Check sheet for the modelled part. Datum: model origin and axes. Units: mm. A direction names the side the tool comes from. Give positions to 0.01 mm unless a question says otherwise; leave off trailing zeros. Write each loop counter-clockwise with the first axis right and the second up, starting at its lowest first coordinate (ties: lowest second). Pieces come first, ordered by that corner, then holes. Notation, with made-up numbers: M 27.25,-29 L 41.25,-29 A17 ccw 41.25,-16 Z; hole C 63.5,81 d4. An arc over 180 degrees is marked long. Write item = value, one per line. Start each with the question number.
1) Sectioned sample at B-B, the plane y = 12. Record the cut outline in (x, z).
2) Set-up check for faces 1 (the face through (-19, 23, 0)), 2 (the face through (-19, -21, -3)), 3 (the face through (-19, -22.5, -3.5)): record each of +Z, -Z, +X, -X, +Y, -Y from which the full face is reachable in a straight line by a thin tool's end or side.
3) Sectioned sample at A-A, the plane x = -19. Record the cut outline in (y, z), then the cut area to 3 significant figures.
4) Sectioned sample at D-D, the plane z = -11. Record the cut outline in (x, y).
5) Sectioned sample at C-C, the plane z = -6.5. Record the cut outline in (x, y), then the cut area to 3 significant figures.
6) Draft check along Y on faces 4 (the face through (-24, 24, -12)), 5 (the face through (-24, -24, -12)), 6 (the face through (-19, -23, 0)), 7 (the face through (-19, 21, -3)). Enter one of: pulls with the +Y half, pulls with the -Y half, needs draft (parallel to the pull), parting line crosses it, or undercut.
7) Scan lines: L1, parallel to X at y = 6, z = -8.5; L2, parallel to Y at x = -20.75, z = -5.5. Record each from-to range of solid material in increasing order.
8) Gauge pin test, flat ends, axial feed: pin 1 (2 mm diameter, centred on y = -16.5, z = -7.5, fed in from +X); pin 2 (0.9 mm diameter, centred on x = -19, y = 22.5, fed in from +Z). Record the tip position at first contact, or that the pin passes through.
from build123d import *

# Parameters (mm, degrees)
SKETCH010_W       = 6
SKETCH010_H       = 48
PAD004_DEPTH      = 6
PAD004_DEPTH_BACK = 30
PAD005_DEPTH      = 3


with BuildPart() as part:
    # Sketch010 (on Face1 of Binder007) → Pad004 (new body, two sides)
    with BuildSketch(Plane.XY) as pad004_sk:
        with Locations((-24, 0)):
            Rectangle(SKETCH010_W, SKETCH010_H)
    extrude(amount=PAD004_DEPTH)
    extrude(pad004_sk.sketch, amount=-PAD004_DEPTH_BACK)

    # Sketch011 (on Face3 of Pad004) → Pad005 (join)
    with BuildSketch(Plane.XZ.offset(24)):
        Polygon((-21, 0), (-21, -7), (-17, 0), align=None)
    pad005 = extrude(amount=-PAD005_DEPTH)

    # Mirrored001: Pad005 across XZ
    add(pad005.mirror(Plane.XZ))


solid = part.part
Data:
q1.outline = M -27,-30 L -21,-30 L -21,6 L -27,6 Z
q2.face_1 = +Z, +X, +Y, -Y
q2.face_2 = +Z, -Z, +X
q2.face_3 = -Z, +X, +Y, -Y
q3.outline = M -24,-3.5 L -21,-3.5 L -21,0 L -24,0 Z; M 21,-3.5 L 24,-3.5 L 24,0 L 21,0 Z
q3.area = 21.0 mm2
q4.outline = M -27,-24 L -21,-24 L -21,24 L -27,24 Z
q5.outline = M -27,-24 L -20.71,-24 L -20.71,-21 L -21,-21 L -21,21 L -20.71,21 L -20.71,24 L -27,24 Z
q5.area = 290 mm2
q6.face_4 = pulls with the +Y half
q6.face_5 = pulls with the -Y half
q6.face_6 = needs draft
q6.face_7 = undercut
q7.L1 = -27 to -21
q7.L2 = -24 to -21, 21 to 24
q8.pin_1 = -21
q8.pin_2 = 0
